Autodesk Inventor part; units mm, degrees
ref_plane "YZ Plane" through (0, 0, 0) normal (1, 0, 0) x (0, 1, 0)
ref_plane "XZ Plane" through (0, 0, 0) normal (0, 1, 0) x (-1, 0, 0)
ref_plane "XY Plane" through (0, 0, 0) normal (0, 0, 1) x (1, 0, 0)
sketch "Sketch1" plane through (0, 0, 0) normal (0, 0, 1) x (1, 0, 0)
  line L0 (0, 0) -> (25.4, 0)
  line L1 (25.4, 0) -> (25.4, 25.4)
  line L2 (25.4, 25.4) -> (0, 25.4)
  line L3 (0, 25.4) -> (0, 0)
  line L4 (3.175, 22.225) -> (22.225, 22.225)
  line L5 (22.225, 22.225) -> (22.225, 3.175)
  line L6 (22.225, 3.175) -> (3.175, 3.175)
  line L7 (3.175, 3.175) -> (3.175, 22.225)
  dimension "d0" = 25.4
  dimension "d1" = 25.4
  dimension "d2" = 3.175
extrude "Extrusion1" add sketch "Sketch1" along normal blind 355.6
sketch "Sketch2" plane through (25.4, 0, 0) normal (1, 0, 0) x (0, 0, -1)
  line L0 (-355.6, 0) -> (-355.6, 25.4)
  line L1 (0, 0) -> (-355.6, 0)
  line L2 (-355.6, 12.7) -> (-342.9, 12.7) construction
  circle A0 centre (-342.9, 12.7) radius 3.302 construction
  circle A1 centre (-317.5, 12.7) radius 3.302
  circle A2 centre (-292.1, 12.7) radius 3.302
  circle A3 centre (-266.7, 12.7) radius 3.302
  circle A4 centre (-241.3, 12.7) radius 3.302
  circle A5 centre (-215.9, 12.7) radius 3.302
  circle A6 centre (-190.5, 12.7) radius 3.302
  circle A7 centre (-165.1, 12.7) radius 3.302
  circle A8 centre (-139.7, 12.7) radius 3.302
  circle A9 centre (-114.3, 12.7) radius 3.302
  circle A10 centre (-88.9, 12.7) radius 3.302
  circle A11 centre (-63.5, 12.7) radius 3.302
  circle A12 centre (-38.1, 12.7) radius 3.302
  circle A13 centre (-12.7, 12.7) radius 3.302
  line L3 (0, 0) -> (0, 25.4)
  circle A14 centre (-342.9, 12.7) radius 3.302
  circle A15 centre (-12.7, 12.7) radius 3.302
  line L4 (-12.7, 12.7) -> (0, 12.7) construction
  dimension "d5" = 12.7
  dimension "d7" = 6.604
  dimension "d10" = 355.6
  dimension "d13" = 25.4
  dimension "d19" = 12.7
  dimension "d20" = 6.604
  dimension "d21" = 6.604
  dimension "d22" = 12.7
extrude "Extrusion2" cut sketch "Sketch2" against normal through all
sketch "Sketch3" plane through (0, 25.4, 0) normal (0, 1, 0) x (1, 0, 0)
  line L0 (25.4, 0) -> (0, 0)
  line L1 (25.4, -355.6) -> (0, -355.6)
  circle A0 centre (12.7, -342.9) radius 3.302
  line L2 (12.7, -355.6) -> (12.7, 0) construction
  circle A1 centre (12.7, -317.5) radius 3.302
  circle A2 centre (12.7, -292.1) radius 3.302
  circle A3 centre (12.7, -266.7) radius 3.302
  circle A4 centre (12.7, -241.3) radius 3.302
  circle A5 centre (12.7, -215.9) radius 3.302
  circle A6 centre (12.7, -190.5) radius 3.302
  circle A7 centre (12.7, -165.1) radius 3.302
  circle A8 centre (12.7, -139.7) radius 3.302
  circle A9 centre (12.7, -114.3) radius 3.302
  circle A10 centre (12.7, -88.9) radius 3.302
  circle A11 centre (12.7, -63.5) radius 3.302
  circle A12 centre (12.7, -38.1) radius 3.302
  circle A13 centre (12.7, -12.7) radius 3.302
  dimension "d23" = 6.604
  dimension "d25" = 12.7
  dimension "d28" = 25.4
extrude "Extrusion3" cut sketch "Sketch3" against normal blind 25.4
equation "\"d20\" = d7"
equation "\"d21\" = d7"
equation "\"d22\" = d19"
properties part number "Chassis Part10 (26x28)" material "Aluminum 6061"
Check sheet for the modelled part. Datum: model origin and axes. Units: mm. Round coordinates to 2 decimals unless told otherwise and drop trailing zeros. Order: outer loops, then holes, each group sorted by start corner. A loop starts at its lowest first (then second) coordinate and runs counter-clockwise, first axis right, second up. Notation, with made-up numbers: M -4,48.5 L 16,48.5 A24 ccw 16,81.5 Z; hole C 58.25,-35 d8. An arc over 180 degrees is marked long. Answer in a Markdown table with one row per item.
(1) Draft check along Z on faces 1 (the flat face through (24, 13, 0)), 2 (the cylindrical face through (11.984, 23.835, 92.123)). Enter one of: +Z half, -Z half, draft (parallel to the pull), parting line (faces both ways), or undercut.
Findings:
| item | result |
|---|---|
| face 1 | -Z half |
| face 2 | undercut |
(2) Gauge pin test, flat end, axial feed: pin 1 (10.5 mm diameter, centred on x = 12.7, z = 190.5, fed in from +Y). Record the tip position at first contact, or that the pin passes through.
Findings:
| item | result |
|---|---|
| pin 1 | stops at y = 25.4 |
(3) Section check A-A on z = 235. Record the boundary of the cut face in (x, y) (3 decimals), plus the area to 3 significant figures.
Findings:
| item | result |
|---|---|
| outline | M 0,0 L 25.4,0 L 25.4,25.4 L 0,25.4 Z; hole M 3.175,3.175 L 22.225,3.175 L 22.225,22.225 L 3.175,22.225 Z |
| area | 282 mm^2 |
(4) Material ranges on line 1 along X through (y, z) = (7.5, 339) (3 decimals); line 2 along X through (y, z) = (23.95, 292.1), recorded low to high. Write a range as from..to.
Findings:
| item | result |
|---|---|
| line 1 | x = 0..3.175, 22.225..25.4 |
| line 2 | x = 0..9.4, 16..25.4 |
